from build123d import *

# Parameters (mm, degrees)
CHAMFER1_SIZE = 0.4


with BuildPart() as part:
    # Sketch1 → Revolve1 (revolve)
    with BuildSketch(Plane(origin=(0, 0, 0), x_dir=(0, 0, -1), z_dir=(1, 0, 0))):
        with BuildLine():
            Line((-4, 3.5), (-13.5274, 3.5))
            Line((-13.5274, 3.5), (-14.2621, 2.7653))
            Line((-14.2621, 2.7653), (-14.2621, 1.7653))
            ThreePointArc((-14.2621, 1.7653), (-13.013844399, 1.248255601), (-12.4968, 0))
            Line((-12.4968, 0), (-3, 0))
            Line((-3, 0), (-3, 0.5))
            Line((-3, 0.5), (-4, 0.5))
            Line((-4, 0.5), (-4, 3.5))
        make_face()
    revolve1 = revolve(axis=Axis((0, 19.017402143, 0), (0, -1, 0)))

    # Mirror1: Revolve1 across plane
    add(revolve1.mirror(Plane.ZX))

    # Chamfer1
    chamfer1_edges = [part.edges().sort_by_distance(p)[0] for p in [
        (0, 3.5, -4),
        (0, -3.5, -4),
    ]]
    chamfer(chamfer1_edges, length=CHAMFER1_SIZE)


solid = part.part
Can you work these out from the model? Positions are in its coordinate system, mm. A direction names the side the tool comes from. Round coordinates to 2 decimals unless told otherwise and drop trailing zeros. Answer in a Markdown table with one row per item. Add a question column.
Q1. I need wall thicknesses on L1, parallel to Z at x = 0, y = -2.3; L2, parallel to Y at x = -9, z = -10.5. Which ranges of each line are inside material? Lowest first, please.
Q2. Which directions (+Z, -Z, +X, -X, +Y, -Y) give clear straight access to the entire face, cutting with the end or side of a thin tool? Please do faces 4 (the cylindrical face through (3.905, -1.818, -0.867)), 5 (the cylindrical face through (3.905, 1.818, -0.867)), 6 (the flat face through (0, 3.5, -6)).
Q3. We'd pull the mould along X, two halves only. Please class faces 1 (the cylindrical face through (0, 0, -3)), 2 (the flat face through (0, -3.5, -6)), 3 (the cylindrical face through (-0.63, 2.26, -14.25)): pulls with the +X half, pulls with the -X half, needs draft (parallel to the pull), parting line crosses it, or undercut.
Q4. For pin 1 Ø2 at (x, y) = (5, -1.5) entering from +Z; pin 2 Ø3 at (y, z) = (1, -7.5) entering from -X; pin 3 Ø5 at (x, z) = (0, 0) entering from +Y; pin 4 Ø4 at (x, y) = (-10, -2.5) entering from -Z, each with a flat end and sliding along its axis, tell me the tip position at first contact or that it passes through.
A:
| question | item | result |
|---|---|---|
| 1 | L1 | -14.26 to -4, 4 to 14.26 |
| 1 | L2 | -3.2 to -1.71, 1.71 to 3.2 |
| 2 | face 4 | -Y |
| 2 | face 5 | +Y |
| 2 | face 6 | +Z, -Z, +X, -X, +Y |
| 3 | face 1 | undercut |
| 3 | face 2 | needs draft |
| 3 | face 3 | parting line crosses it |
| 4 | pin 1 | z = 13.68 |
| 4 | pin 2 | x = -12.84 |
| 4 | pin 3 | through |
| 4 | pin 4 | z = -11.81 |
